Design review of the part shown in the three views and the two pictorial views. Dimensions are in mm from the part's minimum x, y and z. A direction names the side the tool comes from. Round coordinates to 2 decimals unless told otherwise and drop trailing zeros. Order: outer loops, then holes, each group sorted by start corner. A loop starts at its lowest first (then second) coordinate and runs counter-clockwise, first axis right, second up.
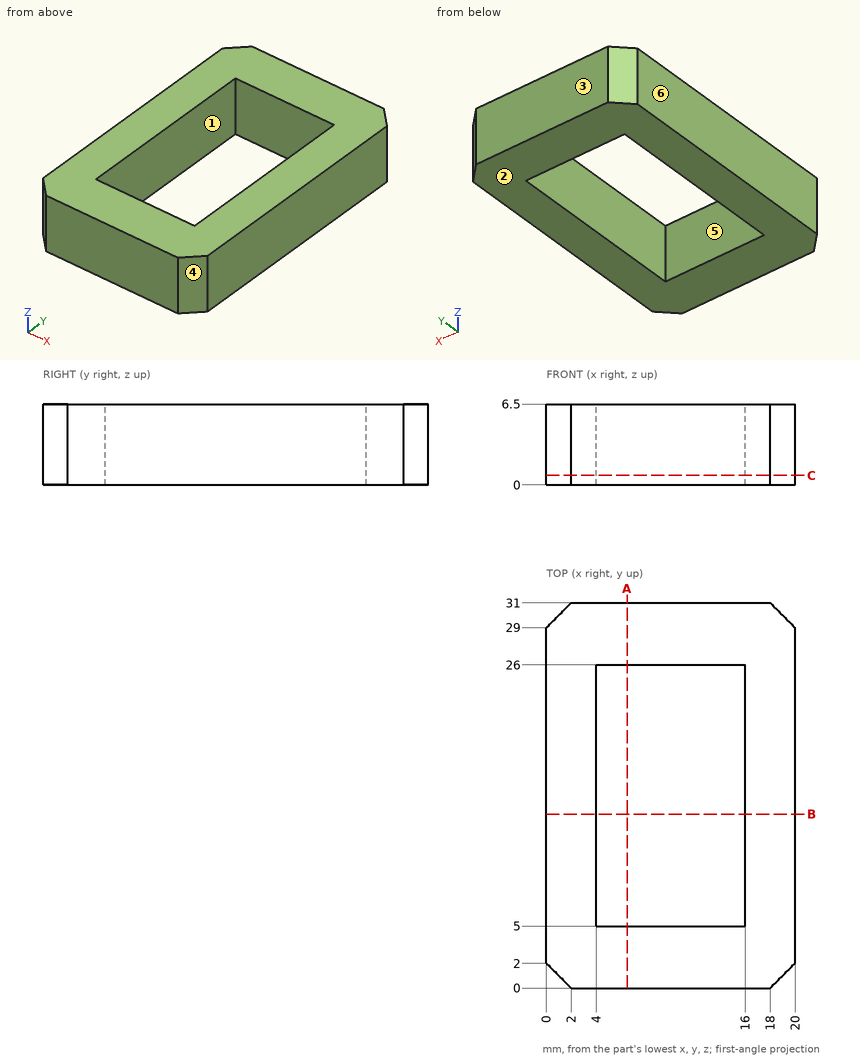
(1) Clearance check with a flat-ended pin moving along its axis: P1, Ø6, axis at x = 9, y = 16.5, coming from the +Z side (3 decimals). State where the tip first meets the part, or that it passes through.
(2) Draft analysis for pull direction X (two halves, no side actions). For the marked faces 3, 4, 5 and 6, state which applies: pulls with the +X half, pulls with the -X half, needs draft (parallel to the pull), parting line crosses it, or undercut.
(3) Tool access review of the marked faces 1 and 2: name each direction out of +Z, -Z, +X, -X, +Y, -Y from which nothing blocks a thin tool from reaching the whole face with its end or side.
(4) Wall thickness on L1, parallel to Y at x = 5.25, z = 1.25; L2, parallel to X at y = 25.5, z = 5.25; L3, parallel to Y at x = 18.5, z = 1.5: over which ranges is each line inside the solid? List them lowest first.
(5) Add section B-B on y = 14. Give the boundary of the cut face in (x, z), plus the area to 3 significant figures.
(6) Add section A-A on x = 6.5. Give the boundary of the cut face in (y, z).
(7) Add section C-C on z = 0.75. Give the boundary of the cut face in (x, y), plus the area to 3 significant figures.
Here are the results:
1. P1: passes through
2. face 3: needs draft
2. face 4: pulls with the +X half
2. face 5: undercut
2. face 6: pulls with the -X half
3. face 1: +Z, -Z
3. face 2: -Z, +X, -X, +Y, -Y
4. L1: y = 0 to 5, 26 to 31
4. L2: x = 0 to 4, 16 to 20
4. L3: y = 0.5 to 30.5
5. outline: (0, 0) - (4, 0) - (4, 6.5) - (0, 6.5) - close; (16, 0) - (20, 0) - (20, 6.5) - (16, 6.5) - close
5. area: 52.0 mm2
6. outline: (0, 0) - (5, 0) - (5, 6.5) - (0, 6.5) - close; (26, 0) - (31, 0) - (31, 6.5) - (26, 6.5) - close
7. outline: (0, 2) - (2, 0) - (18, 0) - (20, 2) - (20, 29) - (18, 31) - (2, 31) - (0, 29) - close; hole (4, 5) - (16, 5) - (16, 26) - (4, 26) - close
7. area: 360 mm2
